```python
from build123d import *

# Parameters (mm, degrees)
RESSALTO_EXTRUS_O1_DEPTH = 2000
CORTE_EXTRUS_O1_DEPTH    = 2001.299713949
CORTE_EXTRUS_O2_DEPTH    = 2001.299713949
CORTE_EXTRUS_O3_DEPTH    = 2001.299713949
CORTE_EXTRUS_O4_DEPTH    = 2001.299713949
CORTE_EXTRUS_O5_DEPTH    = 2001.299713949
FURO1_D                  = 6.27
FURO1_DEPTH              = 17.276941944


with BuildPart() as part:
    # Esboço1 → Ressalto-extrusão1 (new body)
    with BuildSketch(Plane.XZ):
        Polygon((-21.925, -26.8), (21.925, -26.8), (21.925, -22.1), (9.425, -22.1), (3.8, -9.249864864), (0, -10.810968821), (-3.8, -9.249864864), (-9.425, -22.1), (-21.925, -22.1), align=None)
    extrude(amount=-RESSALTO_EXTRUS_O1_DEPTH)

    # Esboço2 → Corte-extrusão1 (cut, through all)
    with BuildSketch(Plane(origin=(0, 2000, 0), x_dir=(-1, 0, 0), z_dir=(0, 1, 0))):
        Polygon((-7.925, -26.8), (7.925, -26.8), (4.5, -20.3), (0.5, -20.3), (0, -19.8), (-0.5, -20.3), (-4.5, -20.3), align=None)
    extrude(amount=-CORTE_EXTRUS_O1_DEPTH, mode=Mode.SUBTRACT)

    # Esboço3 → Corte-extrusão2 (cut, through all)
    with BuildSketch(Plane(origin=(0, 2000, 0), x_dir=(-1, 0, 0), z_dir=(0, 1, 0))):
        Polygon((-15.175, -26.8), (-15.675, -26.3), (-16.175, -26.8), align=None)
    extrude(amount=-CORTE_EXTRUS_O2_DEPTH, mode=Mode.SUBTRACT)

    # Esboço4 → Corte-extrusão3 (cut, through all)
    with BuildSketch(Plane(origin=(0, 2000, 0), x_dir=(-1, 0, 0), z_dir=(0, 1, 0))):
        Polygon((-15.175, -22.1), (-16.175, -22.1), (-15.675, -22.6), align=None)
    extrude(amount=-CORTE_EXTRUS_O3_DEPTH, mode=Mode.SUBTRACT)

    # Esboço5 → Corte-extrusão4 (cut, through all)
    with BuildSketch(Plane(origin=(0, 2000, 0), x_dir=(-1, 0, 0), z_dir=(0, 1, 0))):
        Polygon((16.175, -22.1), (15.175, -22.1), (15.675, -22.6), align=None)
    extrude(amount=-CORTE_EXTRUS_O4_DEPTH, mode=Mode.SUBTRACT)

    # Esboço6 → Corte-extrusão5 (cut, through all)
    with BuildSketch(Plane(origin=(0, 2000, 0), x_dir=(-1, 0, 0), z_dir=(0, 1, 0))):
        Polygon((15.175, -26.8), (16.175, -26.8), (15.675, -26.3), align=None)
    extrude(amount=-CORTE_EXTRUS_O5_DEPTH, mode=Mode.SUBTRACT)

    # Esboço7 → Corte-Revolução1 (revolve, cut)
    with BuildSketch(Plane.XZ.offset(-325), mode=Mode.PRIVATE) as corte_revolu_o1_sk:
        Polygon((19.775, -22.1), (15.675, -22.1), (15.675, -26.8), (18.81, -26.8), (18.81, -23.065), align=None)
    revolve(corte_revolu_o1_sk.sketch.rotate(Axis((15.675, 325, -22.1), (0, 0, -1)), 180), axis=Axis((15.675, 325, -22.1), (0, 0, -1)), mode=Mode.SUBTRACT)

    # Esboço8 → Corte-Revolução2 (revolve, cut)
    with BuildSketch(Plane.XZ.offset(-475), mode=Mode.PRIVATE) as corte_revolu_o2_sk:
        Polygon((19.775, -22.1), (15.675, -22.1), (15.675, -26.8), (18.81, -26.8), (18.81, -23.065), align=None)
    revolve(corte_revolu_o2_sk.sketch.rotate(Axis((15.675, 475, -22.1), (0, 0, -1)), 180), axis=Axis((15.675, 475, -22.1), (0, 0, -1)), mode=Mode.SUBTRACT)

    # Esboço9 → Corte-Revolução3 (revolve, cut)
    with BuildSketch(Plane.XZ.offset(-25), mode=Mode.PRIVATE) as corte_revolu_o3_sk:
        Polygon((19.775, -22.1), (15.675, -22.1), (15.675, -26.8), (18.81, -26.8), (18.81, -23.065), align=None)
    revolve(corte_revolu_o3_sk.sketch.rotate(Axis((15.675, 25, -22.1), (0, 0, -1)), 277.004726435), axis=Axis((15.675, 25, -22.1), (0, 0, -1)), mode=Mode.SUBTRACT)

    # Esboço10 → Corte-Revolução4 (revolve, cut)
    with BuildSketch(Plane.XZ.offset(-175), mode=Mode.PRIVATE) as corte_revolu_o4_sk:
        Polygon((19.775, -22.1), (15.675, -22.1), (15.675, -26.8), (18.81, -26.8), (18.81, -23.065), align=None)
    revolve(corte_revolu_o4_sk.sketch.rotate(Axis((15.675, 175, -22.1), (0, 0, -1)), 180), axis=Axis((15.675, 175, -22.1), (0, 0, -1)), mode=Mode.SUBTRACT)

    # Esboço11 → Corte-Revolução5 (revolve, cut)
    with BuildSketch(Plane.XZ.offset(-175), mode=Mode.PRIVATE) as corte_revolu_o5_sk:
        Polygon((-11.575, -22.1), (-15.675, -22.1), (-15.675, -26.8), (-12.54, -26.8), (-12.54, -23.065), align=None)
    revolve(corte_revolu_o5_sk.sketch.rotate(Axis((-15.675, 175, -22.1), (0, 0, -1)), 277.004726436), axis=Axis((-15.675, 175, -22.1), (0, 0, -1)), mode=Mode.SUBTRACT)

    # Esboço12 → Corte-Revolução6 (revolve, cut)
    with BuildSketch(Plane.XZ.offset(-325), mode=Mode.PRIVATE) as corte_revolu_o6_sk:
        Polygon((-11.575, -22.1), (-15.675, -22.1), (-15.675, -26.8), (-12.54, -26.8), (-12.54, -23.065), align=None)
    revolve(corte_revolu_o6_sk.sketch.rotate(Axis((-15.675, 325, -22.1), (0, 0, -1)), 277.004726436), axis=Axis((-15.675, 325, -22.1), (0, 0, -1)), mode=Mode.SUBTRACT)

    # Esboço13 → Corte-Revolução7 (revolve, cut)
    with BuildSketch(Plane.XZ.offset(-475), mode=Mode.PRIVATE) as corte_revolu_o7_sk:
        Polygon((-11.575, -22.1), (-15.675, -22.1), (-15.675, -26.8), (-12.54, -26.8), (-12.54, -23.065), align=None)
    revolve(corte_revolu_o7_sk.sketch.rotate(Axis((-15.675, 475, -22.1), (0, 0, -1)), 277.004726436), axis=Axis((-15.675, 475, -22.1), (0, 0, -1)), mode=Mode.SUBTRACT)

    # Esboço14 → Corte-Revolução8 (revolve, cut)
    with BuildSketch(Plane.XZ.offset(-25), mode=Mode.PRIVATE) as corte_revolu_o8_sk:
        Polygon((-11.575, -22.1), (-15.675, -22.1), (-15.675, -26.8), (-12.54, -26.8), (-12.54, -23.065), align=None)
    revolve(corte_revolu_o8_sk.sketch.rotate(Axis((-15.675, 25, -22.1), (0, 0, -1)), 277.004726436), axis=Axis((-15.675, 25, -22.1), (0, 0, -1)), mode=Mode.SUBTRACT)

    # Furo1
    with Locations(Plane.XY.offset(-9.523058056)):
        with Locations((0, 175), (0, 25), (0, 475), (0, 325)):
            Hole(FURO1_D / 2, depth=FURO1_DEPTH)


solid = part.part
```
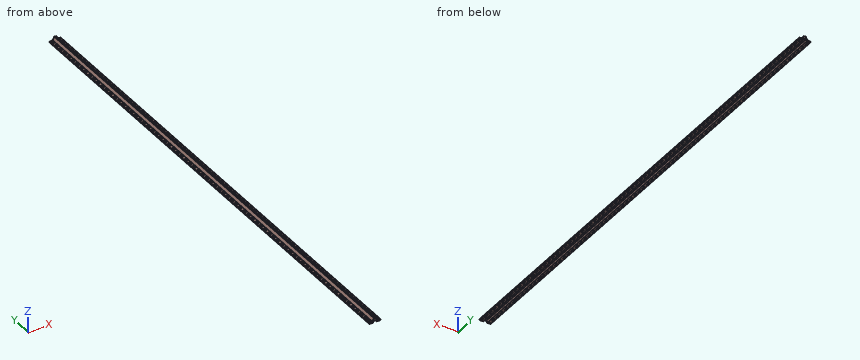
Geometry check sheet. Reference: the model listing, model coordinates, mm. Coordinates: 2 decimals unless noted, no trailing zeros. Order: outer loops, then holes, each group sorted by start corner. A loop starts at its lowest first (then second) coordinate and runs counter-clockwise, first axis right, second up. Notation, with made-up numbers: (34.25, 22.25) - (40.25, 22.25) arc R17 cw to (40.25, 31.25) - close; hole circle Ø9 at (43.25, 82). An arc over 180 degrees is marked (long way). Use one line per item in the form item = value.
1. Gauge pin test, flat ends, axial feed: pin 1 (7 mm diameter, centred on x = 0, y = 475, fed in from +Z); pin 2 (4.5 mm diameter, centred on x = 2.5, y = 1353.5, fed in from -Z); pin 3 (1.7 mm diameter, centred on x = -18, y = 1463.5, fed in from +Z). Record the tip position at first contact, or that the pin passes through.
Here are the results:
pin_1 = -9.37
pin_2 = -20.77
pin_3 = -22.1
2. Section check A-A (y = 1739). Record the boundary of the cut face in (x, z) (3 decimals), then the cut area to 3 significant figures.
Here are the results:
outline = (-21.925, -26.8) - (-16.175, -26.8) - (-15.675, -26.3) - (-15.175, -26.8) - (-7.925, -26.8) - (-4.5, -20.3) - (-0.5, -20.3) - (0, -19.8) - (0.5, -20.3) - (4.5, -20.3) - (7.925, -26.8) - (15.175, -26.8) - (15.675, -26.3) - (16.175, -26.8) - (21.925, -26.8) - (21.925, -22.1) - (16.175, -22.1) - (15.675, -22.6) - (15.175, -22.1) - (9.425, -22.1) - (3.8, -9.25) - (0, -10.811) - (-3.8, -9.25) - (-9.425, -22.1) - (-15.175, -22.1) - (-15.675, -22.6) - (-16.175, -22.1) - (-21.925, -22.1) - close
area = 288 mm²
3. Scan lines: line 1 (Y direction, x = 0, z = -16.25) (3 decimals); line 2 (Y direction, x = -2, z = -17.5); line 3 (X direction, y = 475, z = -24.3) (3 decimals). Record each from-to range of solid material in increasing order.
Here are the results:
line_1 = 0 to 21.865, 28.135 to 171.865, 178.135 to 321.865, 328.135 to 471.865, 478.135 to 2000
line_2 = 0 to 22.59, 27.41 to 172.59, 177.41 to 322.59, 327.41 to 472.59, 477.41 to 2000
line_3 = -21.925 to -18.81, -12.54 to -6.608, 6.608 to 12.54, 18.81 to 21.925
